Input: part model. Units: mm. Frame: model coordinates. A direction names the side the tool comes from. Coordinates: 2 decimals unless noted, no trailing zeros. Loops run counter-clockwise (first coordinate to the right, second up) from the corner with the lowest first, then second, coordinate; pieces in that order, holes last. Notation, with made-up numbers: (14.5, 15) - (50.5, 15) arc R32 ccw to (50.5, 50) - close; hole circle Ø4 at (83, 46). An arc over 180 degrees is marked (long way). Answer as CSV lines item,"result". Start each with the question number.
```python
from build123d import *

# Parameters (mm, degrees)
SKETCH1_W           = 76.2
SKETCH1_H           = 76.2
BOSS_EXTRUDE1_DEPTH = 3.175
SKETCH2_W           = 69.79412
SKETCH2_H           = 69.79412
SKETCH2_W_2         = 57.09412
SKETCH2_H_2         = 57.09412
BOSS_EXTRUDE2_DEPTH = 9.525
FILLET1_R           = 4.7625


with BuildPart() as part:
    # Sketch1 → Boss-Extrude1 (new body)
    with BuildSketch(Plane(origin=(0, 0, 0), x_dir=(1, 0, 0), z_dir=(0, 1, 0))):
        Rectangle(SKETCH1_W, SKETCH1_H)
    extrude(amount=BOSS_EXTRUDE1_DEPTH)

    # Sketch2 → Boss-Extrude2 (add)
    with BuildSketch(Plane(origin=(0, 3.175, 0), x_dir=(1, 0, 0), z_dir=(0, 1, 0))):
        Rectangle(SKETCH2_W, SKETCH2_H)
        Rectangle(SKETCH2_W_2, SKETCH2_H_2, mode=Mode.SUBTRACT)
    extrude(amount=BOSS_EXTRUDE2_DEPTH)

    # Fillet1
    fillet1_edges = [part.edges().sort_by_distance(p)[0] for p in [
        (-28.54706, 7.9375, 28.54706),
        (28.54706, 7.9375, 28.54706),
        (28.54706, 7.9375, -28.54706),
        (-28.54706, 7.9375, -28.54706),
    ]]
    fillet(fillet1_edges, radius=FILLET1_R)

    # Sketch9 → #6-32 Tapped Hole2 (revolve, cut)
    with BuildSketch(Plane(origin=(34.89706, 7.9375, 12.7), x_dir=(0, 0, -1), z_dir=(0, 1, 0))):
        Polygon((0, 0), (0, 11.98869403), (1.35255, 11.176), (1.35255, 0), align=None)
    f_6_32_tapped_hole2 = revolve(axis=Axis((41.24706, 7.9375, 12.7), (-1, 0, 0)), mode=Mode.SUBTRACT)

    # Mirror1: #6-32 Tapped Hole2 across plane
    add(f_6_32_tapped_hole2.mirror(Plane.XY), mode=Mode.SUBTRACT)

    # Mirror2: #6-32 Tapped Hole2 across plane
    add(f_6_32_tapped_hole2.mirror(Plane(origin=(0, 0, 0), x_dir=(0, 0, 1), z_dir=(1, 0, 0))), mode=Mode.SUBTRACT)

    # Mirror2 copy 1 sketch → Mirror2 copy 1 (revolve, cut)
    with BuildSketch(Plane(origin=(-34.89706, 7.9375, -12.7), x_dir=(0, 0, 1), z_dir=(0, 1, 0))):
        Polygon((0, 0), (0, 11.98869403), (1.35255, 11.176), (1.35255, 0), align=None)
    revolve(axis=Axis((-41.24706, 7.9375, -12.7), (1, 0, 0)), mode=Mode.SUBTRACT)


solid = part.part
```
Item 1: Material intervals for probe 1 along X at (y, z) = (8.5, 6); probe 2 along Y at (x, z) = (32.75, -12.7), sorted ascending.
Item 2: Set-up query: faces 4 (the flat face through (0, 8, 34.897)), 5 (the flat face through (-28.547, 8, 0)), 6 (the flat face through (0, 8, -34.897)). Return all of +Z, -Z, +X, -X, +Y, -Y with unobstructed straight access to the full face (end or side cutting, diameter ignored); none if empty.
Item 3: Contact query for flat-ended pins moving along their axis: P1, Ø10, axis at x = -20.5, z = 19, coming from the -Y side; P2, Ø17, axis at x = 5, z = -13, coming from the +Y side (3 decimals); P3, Ø1, axis at x = -4, y = 8, coming from the +Z side; P4, Ø5, axis at y = 6, z = 23, coming from the +X side. Output: stop coordinate, or through.
Item 4: Section query B-B, the plane x = 20. Output: boundary loops of the cut face in (y, z) (3 decimals).
Item 5: Section query D-D, the plane z = -13. Output: boundary loops of the cut face in (x, y) (3 decimals).
Item 6: Draft query along X for faces 1 (the cylindrical face through (31.8, 6.6, 12.9)), 2 (the flat face through (-38.1, 2, 1)), 3 (the cylindrical face through (27.115, 8.004, 27.189)). Return one class per face: pulls with the +X half, pulls with the -X half, needs draft (parallel to the pull), parting line crosses it, or undercut.
Item 7: Section query C-C, the plane z = 26.5. Output: boundary loops of the cut face in (x, y) (3 decimals).
Item 8: Section query A-A, the plane z = 12.7. Output: boundary loops of the cut face in (x, y) (3 decimals).
Response values:
1,probe 1,"x = -34.9 to -28.55, 28.55 to 34.9"
1,probe 2,"y = 0 to 6.58, 9.29 to 12.7"
2,face 4,"+Z, +X, -X, +Y"
2,face 5,"+Y"
2,face 6,"-Z, +X, -X, +Y"
3,P1,"stops at y = 0"
3,P2,"stops at y = 3.175"
3,P3,"stops at z = 34.9"
3,P4,"stops at x = 34.9"
4,outline,"(0, -38.1) - (3.175, -38.1) - (3.175, -34.897) - (12.7, -34.897) - (12.7, -28.547) - (3.175, -28.547) - (3.175, 28.547) - (12.7, 28.547) - (12.7, 34.897) - (3.175, 34.897) - (3.175, 38.1) - (0, 38.1) - close"
5,outline,"(-38.1, 0) - (38.1, 0) - (38.1, 3.175) - (34.897, 3.175) - (34.897, 6.619) - (28.547, 6.619) - (28.547, 3.175) - (-28.547, 3.175) - (-28.547, 6.619) - (-34.897, 6.619) - (-34.897, 3.175) - (-38.1, 3.175) - close; (-34.897, 9.256) - (-28.547, 9.256) - (-28.547, 12.7) - (-34.897, 12.7) - close; (28.547, 9.256) - (34.897, 9.256) - (34.897, 12.7) - (28.547, 12.7) - close"
6,face 1,"needs draft"
6,face 2,"pulls with the -X half"
6,face 3,"undercut"
7,outline,"(-38.1, 0) - (38.1, 0) - (38.1, 3.175) - (34.897, 3.175) - (34.897, 12.7) - (27.697, 12.7) - (27.697, 3.175) - (-27.697, 3.175) - (-27.697, 12.7) - (-34.897, 12.7) - (-34.897, 3.175) - (-38.1, 3.175) - close"
8,outline,"(-38.1, 0) - (38.1, 0) - (38.1, 3.175) - (34.897, 3.175) - (34.897, 6.585) - (28.547, 6.585) - (28.547, 3.175) - (-28.547, 3.175) - (-28.547, 6.585) - (-34.897, 6.585) - (-34.897, 3.175) - (-38.1, 3.175) - close; (-34.897, 9.29) - (-28.547, 9.29) - (-28.547, 12.7) - (-34.897, 12.7) - close; (28.547, 9.29) - (34.897, 9.29) - (34.897, 12.7) - (28.547, 12.7) - close"
